Part model, mm, in its own coordinate system. Give positions to 0.01 mm unless a question says otherwise; leave off trailing zeros. Write each loop counter-clockwise with the first axis right and the second up, starting at its lowest first coordinate (ties: lowest second). Pieces come first, ordered by that corner, then holes.
```python
from build123d import *

# Parameters (mm, degrees)
SKETCH1_W           = 600
SKETCH1_H           = 15
SKETCH1_R           = 4.85
BOSS_EXTRUDE1_DEPTH = 5


with BuildPart() as part:
    # Sketch1 → Boss-Extrude1 (new body)
    with BuildSketch(Plane.XY):
        with Locations((300, -7.5)):
            Rectangle(SKETCH1_W, SKETCH1_H)
        with Locations((6.5, -7.5)):
            Circle(SKETCH1_R, mode=Mode.SUBTRACT)
        with Locations((593.5, -7.5)):
            Circle(SKETCH1_R, mode=Mode.SUBTRACT)
    extrude(amount=-BOSS_EXTRUDE1_DEPTH)


solid = part.part
```
1) Saw through at C-C, the plane z = -1.5. Write the cut outline in (x, y), then the cut area to 3 significant figures.
Answers follow:
outline: (0, -15) - (600, -15) - (600, 0) - (0, 0) - close; hole circle Ø9.7 at (6.5, -7.5); hole circle Ø9.7 at (593.5, -7.5)
area: 8,850 mm2
2) Pin check, flat tip, straight feed: pin 1 Ø1.5 at (y, z) = (-12, -0.5) entering from -X. Stop position of the tip, or through.
Answers follow:
pin 1: stops at x = 0
3) Two-plate mould, pull along Y, no slides. Class faces 1 (the face through (588.655, -7.287, -2.465)), 2 (the face through (296, -7, -5)): +Y half, -Y half, draft (parallel to the pull), parting line (faces both ways), or undercut.
Answers follow:
face 1: undercut
face 2: draft
4) Saw through at A-A, the plane x = 6.5. Write the cut outline in (y, z), then the cut area to 3 significant figures.
Answers follow:
outline: (-15, -5) - (-12.35, -5) - (-12.35, 0) - (-15, 0) - close; (-2.65, -5) - (0, -5) - (0, 0) - (-2.65, 0) - close
area: 26.5 mm2
5) Wall check: L1, parallel to X at y = -8.25, z = -0.4; L2, parallel to Y at x = 6.5, z = -2.2; L3, parallel to X at y = -4, z = -3.3. Give the ranges that are in metal, low to high.
Answers follow:
L1: x = 0 to 1.71, 11.29 to 588.71, 598.29 to 600
L2: y = -15 to -12.35, -2.65 to 0
L3: x = 0 to 3.14, 9.86 to 590.14, 596.86 to 600
6) Saw through at B-B, the plane y = -7.5. Write the cut outline in (x, z).
Answers follow:
outline: (0, -5) - (1.65, -5) - (1.65, 0) - (0, 0) - close; (11.35, -5) - (588.65, -5) - (588.65, 0) - (11.35, 0) - close; (598.35, -5) - (600, -5) - (600, 0) - (598.35, 0) - close
